Input: part model. Units: mm. Frame: model coordinates. A direction names the side the tool comes from. Coordinates: 2 decimals unless noted, no trailing zeros. Loops run counter-clockwise (first coordinate to the right, second up) from the corner with the lowest first, then second, coordinate; pieces in that order, holes last. Notation, with made-up numbers: (53.5, 6) - (103.5, 6) arc R26 cw to (103.5, 28) - close; hole circle Ø1 at (84, 78.25). An arc over 180 degrees is marked (long way). Write item = value, one per line. Start each with the question number.
from build123d import *

# Parameters (mm, degrees)
SKETCH1_W           = 47.498
SKETCH1_H           = 36.6014
BOSS_EXTRUDE1_DEPTH = 2.667
SKETCH3_W           = 5.334
SKETCH3_H           = 7.32028
BOSS_EXTRUDE3_DEPTH = 5.334
SKETCH5_W           = 15.832666666
SKETCH5_H           = 5.334
BOSS_EXTRUDE4_DEPTH = 5.334
SKETCH6_R           = 1.27
SKETCH6_R_2         = 5.8801
CUT_EXTRUDE1_DEPTH  = 38.853289013


with BuildPart() as part:
    # Sketch1 → Boss-Extrude1 (new, symmetric)
    with BuildSketch(Plane.XY):
        Rectangle(SKETCH1_W, SKETCH1_H)
    extrude(amount=BOSS_EXTRUDE1_DEPTH, both=True)

    # Sketch3 → Boss-Extrude3 (add)
    with BuildSketch(Plane.XY.offset(2.667)):
        with Locations((-26.416, 7.32028)):
            Rectangle(SKETCH3_W, SKETCH3_H)
        with Locations((-26.416, -7.32028)):
            Rectangle(SKETCH3_W, SKETCH3_H)
        with Locations((26.416, -7.32028)):
            Rectangle(SKETCH3_W, SKETCH3_H)
        with Locations((26.416, 7.32028)):
            Rectangle(SKETCH3_W, SKETCH3_H)
    extrude(amount=-BOSS_EXTRUDE3_DEPTH)

    # Sketch5 → Boss-Extrude4 (add)
    with BuildSketch(Plane.XY.offset(2.667)):
        with Locations((0, -20.9677)):
            Rectangle(SKETCH5_W, SKETCH5_H)
        with Locations((0, 20.9677)):
            Rectangle(SKETCH5_W, SKETCH5_H)
    extrude(amount=-BOSS_EXTRUDE4_DEPTH)

    # Sketch6 → Cut-Extrude1 (cut, through all)
    with BuildSketch(Plane(origin=(0, 0, -2.667), x_dir=(-1, 0, 0), z_dir=(0, 0, -1))):
        with Locations((-15.24, -0.0762)):
            Circle(SKETCH6_R)
        with Locations((-7.62, -13.274427096)):
            Circle(SKETCH6_R)
        with Locations((15.24, -0.0762)):
            Circle(SKETCH6_R)
        with Locations((-7.61999995, 13.122027183)):
            Circle(SKETCH6_R)
        with Locations((0, -6.9596)):
            Circle(SKETCH6_R_2)
    extrude(amount=-CUT_EXTRUDE1_DEPTH, mode=Mode.SUBTRACT)


solid = part.part
Item 1: Cut plane C-C on y = -9.5. Return loops of the section in (x, z).
Item 2: Cut plane D-D on y = -20. Return loops of the section in (x, z).
Item 3: Access query for faces 5 (the flat face through (-23.749, 0, 0)), 6 (the flat face through (23.749, 15, 0)), 7 (the flat face through (-26, 10.98, 0)), 8 (the flat face through (23.749, -15, 0)). Directions: +Z, -Z, +X, -X, +Y, -Y. A direction counts if a zero-diameter tool reaches every point of the face in a straight line with its end or side. Return the directions, or none.
Item 4: Pin query (flat end, axial travel): pin 1 (2 mm diameter, centred on x = 23, z = 2, fed in from +Y); pin 2 (1.6 mm diameter, centred on x = 27.5, z = 1, fed in from +Y); pin 3 (2 mm diameter, centred on y = -1, z = -2, fed in from +X). Return the tip coordinate at first contact, or that it passes through.
Item 5: Cut plane B-B on z = 0.75. State how many separate pieces and enclosed holes the cut face has, plus the area to 3 significant figures.
Item 6: Ray query, line 1 (Y direction, x = 7.62, z = -0.5); line 2 (Y direction, x = 0, z = -0.2); line 3 (Y direction, x = -15.24, z = 1.6). Return the intervals inside material, ascending.
Item 7: Cut plane A-A on x = 15.24. Return loops of the section in (y, z), plus the area to 3 significant figures.
Item 8: Pull-direction query (Y, two-part tool) for faces 1 (the flat face through (-26, -3.66, 0)), 2 (the flat face through (-26, -10.98, 0)), 3 (the flat face through (16, 18.301, 0)), 4 (the flat face through (23.749, 0, 0)); classes: pulls with the +Y half, pulls with the -Y half, needs draft (parallel to the pull), parting line crosses it, or undercut.
Recorded:
q1.outline = (-29.08, -2.67) - (-5.3, -2.67) - (-5.3, 2.67) - (-29.08, 2.67) - close; (5.3, -2.67) - (29.08, -2.67) - (29.08, 2.67) - (5.3, 2.67) - close
q2.outline = (-7.92, -2.67) - (7.92, -2.67) - (7.92, 2.67) - (-7.92, 2.67) - close
q3.face_5 = +Z, -Z, -X
q3.face_6 = +Z, -Z, +X, +Y
q3.face_7 = +Z, -Z, -X, +Y
q3.face_8 = +Z, -Z, +X, -Y
q4.pin_1 = 18.3
q4.pin_2 = 10.98
q4.pin_3 = 23.75
q5.separate_pieces = 1
q5.enclosed_holes = 5
q5.area = 1,930 mm²
q6.line_1 = -23.63 to -14.54, -12 to 11.85, 14.39 to 23.63
q6.line_2 = -23.63 to -12.84, -1.08 to 23.63
q6.line_3 = -18.3 to -1.35, 1.19 to 18.3
q7.outline = (-18.3, -2.67) - (-1.35, -2.67) - (-1.35, 2.67) - (-18.3, 2.67) - close; (1.19, -2.67) - (18.3, -2.67) - (18.3, 2.67) - (1.19, 2.67) - close
q7.area = 182 mm²
q8.face_1 = undercut
q8.face_2 = pulls with the -Y half
q8.face_3 = pulls with the +Y half
q8.face_4 = undercut
